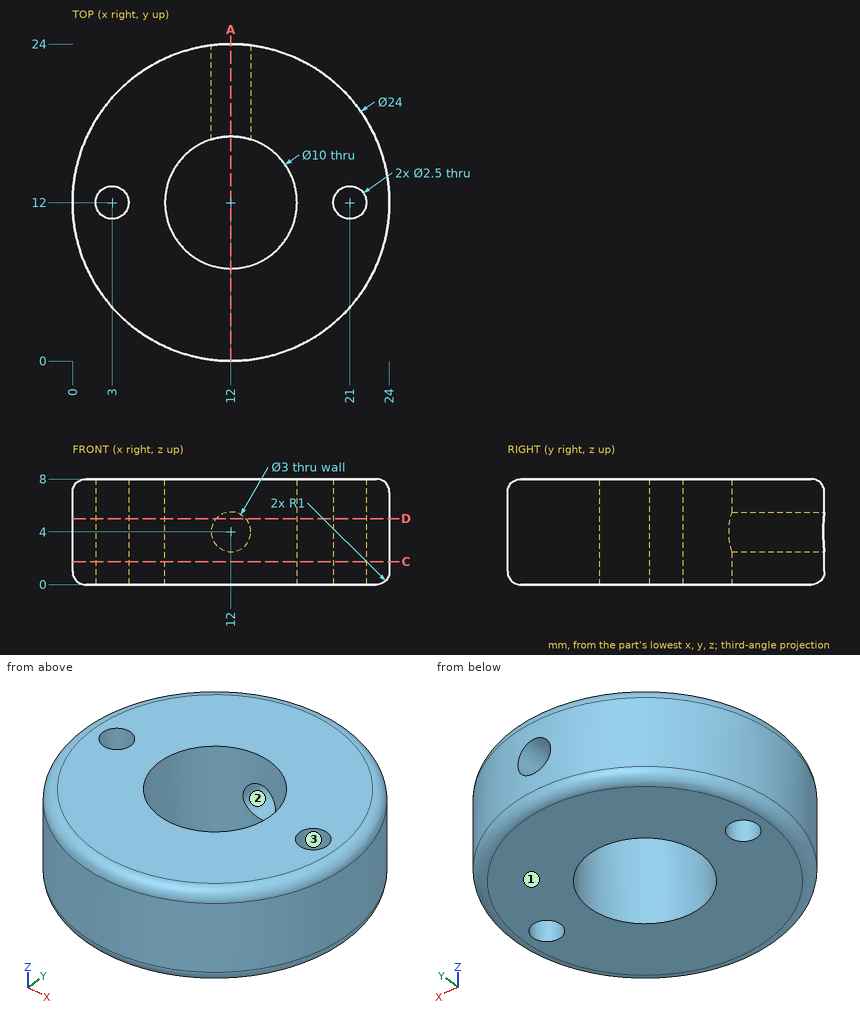
Input: dimensioned drawing with shaded views. Units: mm. Origin: part minimum x, y, z. Coordinates: 2 decimals unless noted, no trailing zeros. Loops run counter-clockwise (first coordinate to the right, second up) from the corner with the lowest first, then second, coordinate; pieces in that order, holes last.
Q1. Contact query for flat-ended pins moving along their axis: pin 1 (3 mm diameter, centred on y = 8.5, z = 3, fed in from +X); pin 2 (1.5 mm diameter, centred on x = 5, z = 5.5, fed in from +Y); pin 3 (2.5 mm diameter, centred on x = 12, z = 4, fed in from +Y). Output: stop coordinate, or through.
Results are:
pin 1: stops at x = 23.83
pin 2: stops at y = 22.24
pin 3: stops at y = 7.16
Q2. Mould query, pull axis Z, two halves, no side actions, for the marked faces 1, 2 and 3. Classes: +Z half, -Z half, draft (parallel to the pull), parting line (faces both ways), or undercut.
Results are:
face 1: -Z half
face 2: undercut
face 3: draft
Q3. Line query: line 1 along Z through (x, y) = (12, 19.5); line 2 along Y through (x, z) = (15.25, 4.5); line 3 along Y through (x, z) = (3.5, 6). Output: solid intervals per line, ascending.
Results are:
line 1: z = 0 to 2.5, 5.5 to 8
line 2: y = 0.45 to 8.2, 15.8 to 23.55
line 3: y = 3.53 to 10.85, 13.15 to 20.47
Q4. Section A-A, the plane x = 12. Give the number of separate pieces and of enclosed holes in the cut face, and give its area (3 significant figures).
Results are:
separate pieces: 3
enclosed holes: 0
area: 90.1 mm2
Q5. Section C-C, the plane z = 1.75. Return the cut outline in (x, y).
Results are:
outline: circle Ø24 at (12, 12); hole circle Ø2.5 at (3, 12); hole circle Ø10 at (12, 12); hole circle Ø2.5 at (21, 12)
Q6. Section D-D, the plane z = 5. Return the cut outline in (x, y).
Results are:
outline: (10.88, 16.87) - (10.88, 23.95) arc R12 ccw (long way) to (13.12, 23.95) - (13.12, 16.87) arc R5 cw (long way) to start; hole circle Ø2.5 at (3, 12); hole circle Ø2.5 at (21, 12)
